from build123d import *

# Parameters (mm, degrees)
SKETCH1_W           = 12.319
SKETCH1_H           = 12.319
BOSS_EXTRUDE1_DEPTH = 7.5692
SKETCH2_W           = 10.3124
SKETCH2_H           = 10.3124
BOSS_EXTRUDE2_DEPTH = 2.286
SKETCH3_R           = 0.6096
BOSS_EXTRUDE5_DEPTH = 1.4986
FILLET2_R           = 0.5
FILLET3_R           = 0.1
SKETCH5_W           = 0.9906
SKETCH5_H           = 0.9906
BOSS_EXTRUDE6_DEPTH = 3.8608
CHAMFER1_SIZE       = 0.1
FILLET4_R           = 0.1
FILLET5_R           = 0.1
FILLET6_R           = 0.1
FILLET7_R           = 0.1


with BuildPart() as part:
    # Sketch1 → Boss-Extrude1 (new body)
    with BuildSketch(Plane.XY):
        Rectangle(SKETCH1_W, SKETCH1_H)
    extrude(amount=BOSS_EXTRUDE1_DEPTH)

    # Sketch2 → Boss-Extrude2 (add)
    with BuildSketch(Plane.XY.offset(7.5692)):
        Rectangle(SKETCH2_W, SKETCH2_H)
    extrude(amount=BOSS_EXTRUDE2_DEPTH)

    # Sketch3 → Boss-Extrude5 (add)
    with BuildSketch(Plane(origin=(0, 0, 0), x_dir=(-1, 0, 0), z_dir=(0, 0, -1))):
        with Locations((-1.2295, 1.2295)):
            Circle(SKETCH3_R)
        with Locations((-3.7695, -1.3105)):
            Circle(SKETCH3_R)
    extrude(amount=BOSS_EXTRUDE5_DEPTH)

    # Fillet2
    fillet2_edges = [part.edges().sort_by_distance(p)[0] for p in [
        (1.8391, 1.2295, -1.4986),
        (4.3791, -1.3105, -1.4986),
    ]]
    fillet(fillet2_edges, radius=FILLET2_R)

    # Fillet3
    fillet3_edges = [part.edges().sort_by_distance(p)[0] for p in [
        (1.8391, 1.2295, 0),
        (4.3791, -1.3105, 0),
    ]]
    fillet(fillet3_edges, radius=FILLET3_R)

    # Sketch5 → Boss-Extrude6 (add)
    with BuildSketch(Plane(origin=(0, 0, 0), x_dir=(-1, 0, 0), z_dir=(0, 0, -1))):
        with Locations((3.8505, -3.8505)):
            Rectangle(SKETCH5_W, SKETCH5_H)
        with Locations((3.8505, 3.7695)):
            Rectangle(SKETCH5_W, SKETCH5_H)
    extrude(amount=BOSS_EXTRUDE6_DEPTH)

    # Chamfer1
    chamfer1_edges = [part.edges().sort_by_distance(p)[0] for p in [
        (-3.8505, -3.3552, -3.8608),
        (-3.3552, -3.8505, -3.8608),
        (-3.8505, -4.3458, -3.8608),
        (-4.3458, -3.8505, -3.8608),
        (-3.3552, 3.7695, -3.8608),
        (-3.8505, 4.2648, -3.8608),
        (-3.8505, 3.2742, -3.8608),
        (-4.3458, 3.7695, -3.8608),
    ]]
    chamfer(chamfer1_edges, length=CHAMFER1_SIZE)

    # Fillet4
    fillet4_edges = [part.edges().sort_by_distance(p)[0] for p in [
        (-3.8505, -4.3458, 0),
        (-4.3458, -3.8505, 0),
        (-3.8505, -3.3552, 0),
        (-3.3552, -3.8505, 0),
        (-3.8505, 3.2742, 0),
        (-4.3458, 3.7695, 0),
        (-3.3552, 3.7695, 0),
        (-3.8505, 4.2648, 0),
    ]]
    fillet(fillet4_edges, radius=FILLET4_R)

    # Fillet5
    fillet5_edges = [part.edges().sort_by_distance(p)[0] for p in [
        (5.1562, 0, 7.5692),
        (0, 5.1562, 7.5692),
        (-5.1562, 0, 7.5692),
        (0, -5.1562, 7.5692),
    ]]
    fillet(fillet5_edges, radius=FILLET5_R)

    # Fillet6
    fillet6_edges = [part.edges().sort_by_distance(p)[0] for p in [
        (-4.381195109, 3.238804891, -0.023670398),
        (-4.381195109, 4.300195109, -0.023670398),
        (-3.319804891, 3.238804891, -0.023670398),
        (-3.319804891, 4.300195109, -0.023670398),
        (-3.319804891, -4.381195109, -0.023670398),
        (-4.381195109, -4.381195109, -0.023670398),
        (-3.319804891, -3.319804891, -0.023670398),
        (-4.381195109, -3.319804891, -0.023670398),
        (-3.3552, -4.3458, -1.9304),
        (-3.3552, -3.3552, -1.9304),
        (-4.3458, -4.3458, -1.9304),
        (-4.3458, -3.3552, -1.9304),
        (-3.3552, 3.2742, -1.9304),
        (-3.3552, 4.2648, -1.9304),
        (-4.3458, 3.2742, -1.9304),
        (-4.3458, 4.2648, -1.9304),
    ]]
    fillet(fillet6_edges, radius=FILLET6_R)

    # Fillet7
    fillet7_edges = [part.edges().sort_by_distance(p)[0] for p in [
        (5.1562, 0, 9.8552),
        (0, 5.1562, 9.8552),
        (-5.1562, 0, 9.8552),
        (0, -5.1562, 9.8552),
    ]]
    fillet(fillet7_edges, radius=FILLET7_R)


solid = part.part
Source: CAD feature listing. Evaluate the final solid. Frame: model axes, mm. A direction names the side the tool comes from. Coordinates: 2 decimals unless noted, no trailing zeros. Order: outer loops, then holes, each group sorted by start corner. A loop starts at its lowest first (then second) coordinate and runs counter-clockwise, first axis right, second up. Notation, with made-up numbers: M 71.25,88.5 L 112.25,88.5 A25 ccw 112.25,105.5 Z; hole C 61,-25.75 d10. An arc over 180 degrees is marked long. Write each question's results on one line, items separated by ' | '. Start each with the question number.
Item 1: Cut plane B-B (x = -3.75). Return loops of the section in (y, z).
Item 2: Cut plane D-D (z = 8.5). Return loops of the section in (x, y).
Item 3: Draft query along Y for faces 1 (the face through (-6, 0, 7.569)), 2 (the face through (0, 6.16, 4)), 3 (the face through (4.38, -1.28, -0.54)). Return one class per face: pulls with the +Y half, pulls with the -Y half, needs draft (parallel to the pull), parting line crosses it, or undercut.
Item 4: Set-up query: faces 4 (the face through (0, 5.156, 9)), 5 (the face through (0, 0, 0)), 6 (the face through (5.156, 0, 9)), 7 (the face through (-5.156, 0, 9)). Return all of +Z, -Z, +X, -X, +Y, -Y with unobstructed straight access to the full face (end or side cutting, diameter ignored); none if empty.
Item 5: Cut plane C-C (y = 2.5). Return loops of the section in (x, z), and give its area (3 significant figures).
Item 6: Cut plane A-A (z = -2.5). Return loops of the section in (x, y).
Item 7: Line query: probe 1 along Z at (x, y) = (-5, -1.75); probe 2 along Z at (x, y) = (5.5, 3.25); probe 3 along Y at (x, z) = (1.25, 8.5). Output: solid intervals per line, ascending.
Item 8: First-contact query: pin 1 Ø3.5 at (x, y) = (-1.5, 2) entering from -Z; pin 2 Ø0.6 at (y, z) = (-2, 9) entering from -X; pin 3 Ø0.9 at (x, z) = (-4, -1) entering from -Y. Flat tips, straight axial feed; report the tip coordinate or a pass-through.
Checked values:
1) outline: M -6.16,0 L -4.45,0 A0.1 cw -4.35,-0.1 L -4.35,-3.76 L -4.25,-3.86 L -3.46,-3.86 L -3.36,-3.76 L -3.36,-0.1 A0.1 cw -3.26,0 L 3.17,0 A0.1 cw 3.27,-0.1 L 3.27,-3.76 L 3.37,-3.86 L 4.16,-3.86 L 4.26,-3.76 L 4.26,-0.1 A0.1 cw 4.36,0 L 6.16,0 L 6.16,7.57 L 5.26,7.57 A0.1 cw 5.16,7.67 L 5.16,9.76 A0.1 ccw 5.06,9.86 L -5.06,9.86 A0.1 ccw -5.16,9.76 L -5.16,7.67 A0.1 cw -5.26,7.57 L -6.16,7.57 Z
2) outline: M -5.16,-5.16 L 5.16,-5.16 L 5.16,5.16 L -5.16,5.16 Z
3) face 1: needs draft | face 2: pulls with the +Y half | face 3: parting line crosses it
4) face 4: +Z, +X, -X, +Y | face 5: -Z | face 6: +Z, +X, +Y, -Y | face 7: +Z, -X, +Y, -Y
5) outline: M -6.16,0 L 6.16,0 L 6.16,7.57 L 5.26,7.57 A0.1 cw 5.16,7.67 L 5.16,9.76 A0.1 ccw 5.06,9.86 L -5.06,9.86 A0.1 ccw -5.16,9.76 L -5.16,7.67 A0.1 cw -5.26,7.57 L -6.16,7.57 Z | area: 117 mm2
6) outline: M -4.35,-4.25 A0.1 ccw -4.25,-4.35 L -3.46,-4.35 A0.1 ccw -3.36,-4.25 L -3.36,-3.46 A0.1 ccw -3.46,-3.36 L -4.25,-3.36 A0.1 ccw -4.35,-3.46 Z; M -4.35,3.37 A0.1 ccw -4.25,3.27 L -3.46,3.27 A0.1 ccw -3.36,3.37 L -3.36,4.16 A0.1 ccw -3.46,4.26 L -4.25,4.26 A0.1 ccw -4.35,4.16 Z
7) probe 1: z = 0 to 9.86 | probe 2: z = 0 to 7.57 | probe 3: y = -5.16 to 5.16
8) pin 1: stops at z = 0 | pin 2: stops at x = -5.16 | pin 3: stops at y = -4.35
